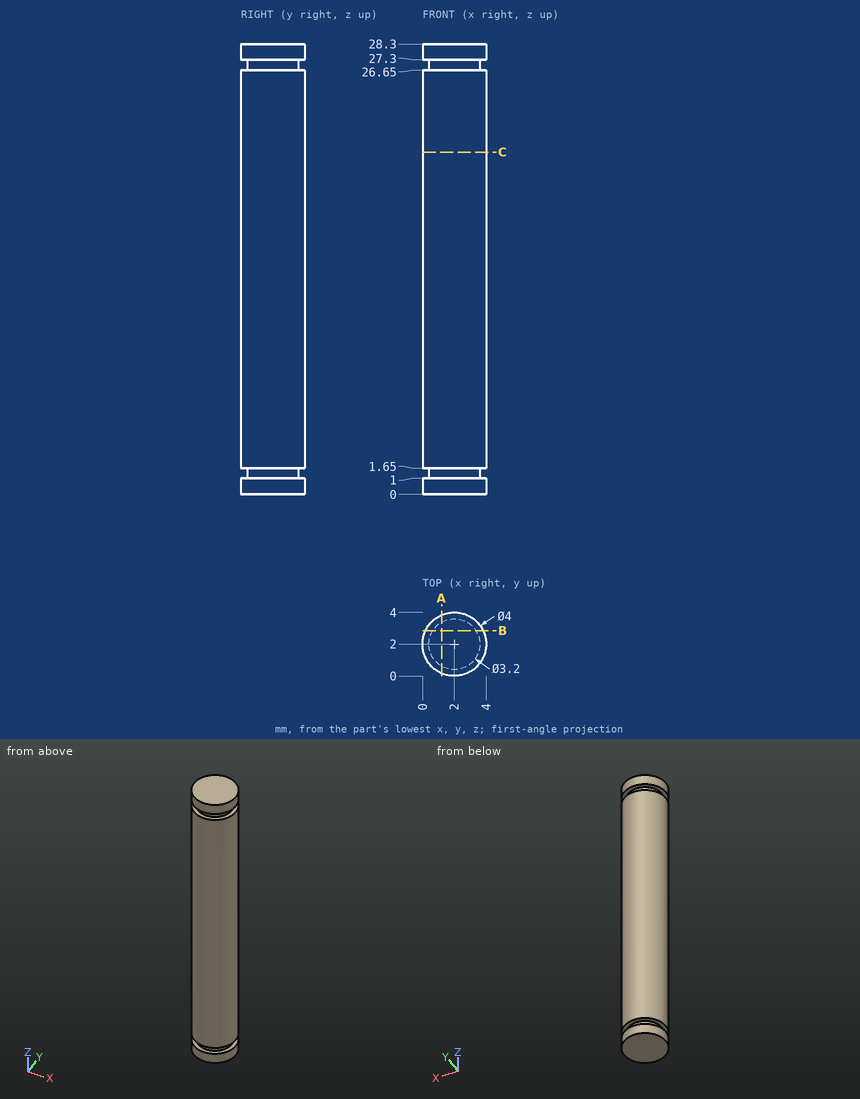
Answer from the drawing. Dimensions are ordinates in mm from the lowest x, y and z of the part. Give positions to 0.01 mm unless a question says otherwise; leave off trailing zeros. Write each loop counter-clockwise with the first axis right and the second up, starting at its lowest first coordinate (ties: lowest second). Pieces come first, ordered by that corner, then holes. Notation, with made-up numbers: (82, 3.25) -> (103, 3.25) arc R23 cw to (103, 26.25) -> close; hole circle Ø3 at (61.5, -16). An arc over 180 degrees is marked (long way). Use a Markdown table: item, result.
(1) Find the intervals of material crossed by probe 1 along Z at (x, y) = (3.85, 2.25); probe 2 along Y at (x, z) = (2.1, 23.5), in increasing order. Write a range as from..to.
Return value:
| item | result |
|---|---|
| probe 1 | 0..1, 1.65..26.65, 27.3..28.3 |
| probe 2 | 0..4 |
(2) Section A-A, the plane x = 1.2 is taken. Determine the outline of the cut face in (y, z), then the cut area to 3 significant figures.
Return value:
| item | result |
|---|---|
| outline | (0.17, 0) -> (3.83, 0) -> (3.83, 1) -> (3.39, 1) -> (3.39, 1.65) -> (3.83, 1.65) -> (3.83, 26.65) -> (3.39, 26.65) -> (3.39, 27.3) -> (3.83, 27.3) -> (3.83, 28.3) -> (0.17, 28.3) -> (0.17, 27.3) -> (0.61, 27.3) -> (0.61, 26.65) -> (0.17, 26.65) -> (0.17, 1.65) -> (0.61, 1.65) -> (0.61, 1) -> (0.17, 1) -> close |
| area | 103 mm2 |
(3) Section B-B, the plane y = 2.85 is taken. Determine the outline of the cut face in (x, z).
Return value:
| item | result |
|---|---|
| outline | (0.19, 0) -> (3.81, 0) -> (3.81, 1) -> (3.36, 1) -> (3.36, 1.65) -> (3.81, 1.65) -> (3.81, 26.65) -> (3.36, 26.65) -> (3.36, 27.3) -> (3.81, 27.3) -> (3.81, 28.3) -> (0.19, 28.3) -> (0.19, 27.3) -> (0.64, 27.3) -> (0.64, 26.65) -> (0.19, 26.65) -> (0.19, 1.65) -> (0.64, 1.65) -> (0.64, 1) -> (0.19, 1) -> close |
(4) Section C-C, the plane z = 21.5 is taken. Determine the outline of the cut face in (x, y).
Return value:
| item | result |
|---|---|
| outline | circle Ø4 at (2, 2) |
